Could you check a few things on this model? Use its own coordinates, in mm. Face numbers are marked on the shaded views. A direction names the side the tool comes from. Give positions to 0.01 mm unless a question says otherwise; leave off trailing zeros. Write each loop counter-clockwise with the first axis right and the second up, starting at its lowest first coordinate (ties: lowest second). Pieces come first, ordered by that corner, then holes. Notation, with made-up numbers: M -18,-3.5 L 33,-3.5 A22 cw 33,3.5 Z; hole C 72,-36.5 d7. An arc over 180 degrees is marked long. Use one line per item in the form item = value.
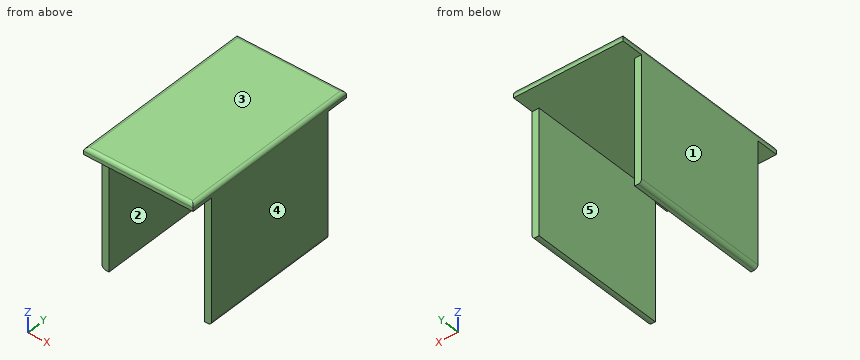
from build123d import *

# Parameters (mm, degrees)
SKETCH006_W  = 10
SKETCH006_H  = 9.5
PAD002_DEPTH = 0.5
SKETCH007_W  = 7.9
SKETCH007_H  = 13.2
PAD003_DEPTH = 0.5
SKETCH008_W  = 10
SKETCH008_H  = 9.5
PAD004_DEPTH = 0.5
FILLET_R     = 0.25


with BuildPart() as part:
    # Sketch006 → Pad002 (new body)
    with BuildSketch(Plane.YZ.offset(3.95)):
        with Locations((0, 4.75)):
            Rectangle(SKETCH006_W, SKETCH006_H)
    extrude(amount=-PAD002_DEPTH)

    # Sketch007 → Pad003 (join)
    with BuildSketch(Plane.XY.offset(9.5)):
        Rectangle(SKETCH007_W, SKETCH007_H)
    extrude(amount=-PAD003_DEPTH)

    # Sketch008 → Pad004 (join)
    with BuildSketch(Plane.YZ.offset(-3.95)):
        with Locations((0, 4.75)):
            Rectangle(SKETCH008_W, SKETCH008_H)
    extrude(amount=PAD004_DEPTH)

    # Fillet
    fillet_edges = [part.edges().sort_by_distance(p)[0] for p in [
        (3.95, 0, 9.5),
        (0, 6.6, 9.5),
        (-3.95, 0, 9.5),
        (0, -6.6, 9.5),
        (3.95, 0, 0),
        (-3.95, 0, 0),
    ]]
    fillet(fillet_edges, radius=FILLET_R)


solid = part.part
1) For pin 1 Ø4 at (x, y) = (-2, -1) entering from -Z; pin 2 Ø2 at (x, y) = (-0.5, 3) entering from -Z, each with a flat end and sliding along its axis, tell me the tip position at first contact or that it passes through.
Checked values:
pin_1 = 0
pin_2 = 9
2) I want a section at B-B, the plane y = -4.5. Please give me the cut outline in (x, z).
Checked values:
outline = M -3.95,0.25 A0.25 ccw -3.7,0 L -3.45,0 L -3.45,9 L 3.45,9 L 3.45,0 L 3.7,0 A0.25 ccw 3.95,0.25 L 3.95,9.25 A0.25 ccw 3.7,9.5 L -3.7,9.5 A0.25 ccw -3.95,9.25 Z
3) If I drill on L1, parallel to X at y = 1.75, z = 7; L2, parallel to Z at x = -2, y = -1, over which ranges is the centre line in solid material (lowest first)?
Checked values:
L1 = -3.95 to -3.45, 3.45 to 3.95
L2 = 9 to 9.5
4) For the marked faces 1 and 2, which set-ups out of +Z, -Z, +X, -X, +Y, -Y let a thin tool reach every point of the face, with its end or its side?
Checked values:
face_1 = +Z, -Z, -X, +Y, -Y
face_2 = -Z, +Y, -Y
5) I want a section at C-C, the plane x = 3. Please give me the cut outline in (y, z), plus the area to 3 significant figures.
Checked values:
outline = M -6.6,9 L 6.6,9 L 6.6,9.25 A0.25 ccw 6.35,9.5 L -6.35,9.5 A0.25 ccw -6.6,9.25 Z
area = 6.57 mm2
6) I want a section at A-A, the plane z = 3.5. Please give me the cut outline in (x, y).
Checked values:
outline = M -3.95,-5 L -3.45,-5 L -3.45,5 L -3.95,5 Z; M 3.45,-5 L 3.95,-5 L 3.95,5 L 3.45,5 Z
7) I want a section at D-D, the plane y = 5.25. Please give me the cut outline in (x, z), plus the area to 3 significant figures.
Checked values:
outline = M -3.95,9 L 3.95,9 L 3.95,9.25 A0.25 ccw 3.7,9.5 L -3.7,9.5 A0.25 ccw -3.95,9.25 Z
area = 3.92 mm2
8) Thinking about a two-plate mould opening in X: for the marked faces 3, 4 and 5, which applies, released by +X, released by -X, zero draft, split by the parting line, or undercut?
Checked values:
face_3 = zero draft
face_4 = released by +X
face_5 = undercut
